```python
from build123d import *

# Parameters (mm, degrees)
F0_W     = 203.2
F0_H     = 76.2
F1_DEPTH = 76.708
F2_W     = 101.6
F2_H     = 38.1
F3_DEPTH = 116.332
F4_R     = 7.5946
F5_DEPTH = 234.95
F6_W     = 176.251258
F6_H     = 58.252844
F7_DEPTH = 93.472


with BuildPart() as f1:
    # F0 (on Front) → F1 (new body)
    with BuildSketch(Plane.XZ):
        with Locations((48.921661, 38.1)):
            Rectangle(F0_W, F0_H)
    extrude(amount=F1_DEPTH)

    # F2 (on Front) → F3 (cut)
    with BuildSketch(Plane.XZ):
        with Locations((49.131309, 57.448106)):
            Rectangle(F2_W, F2_H)
    extrude(amount=F3_DEPTH, mode=Mode.SUBTRACT)

    # F4 (on face) → F5 (cut, symmetric)
    with BuildSketch(Plane(origin=(-52.678339, 0, 0), x_dir=(0, -1, 0), z_dir=(-1, 0, 0))):
        with Locations((40.342383, 40.232584)):
            Circle(F4_R)
    extrude(amount=F5_DEPTH, both=True, mode=Mode.SUBTRACT)

    # F6 (on face) → F7 (cut)
    with BuildSketch(Plane(origin=(0, 0, 0), x_dir=(1, 0, 0), z_dir=(0, 0, -1))):
        with Locations((45.208322, 38.419208)):
            Rectangle(F6_W, F6_H)
    extrude(amount=-F7_DEPTH, mode=Mode.SUBTRACT)


solid = f1.part
```
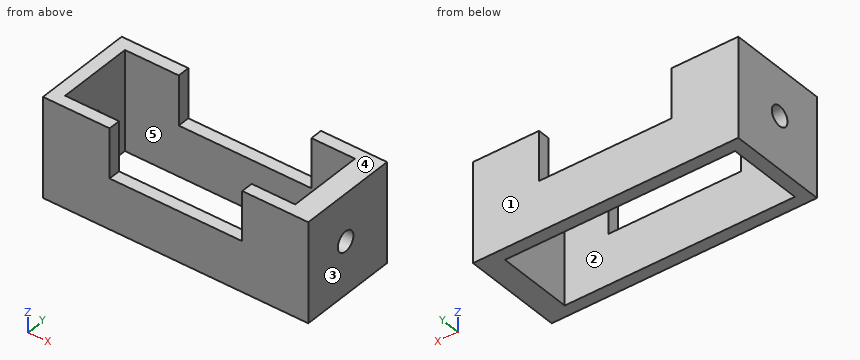
Can you work these out from the model? Positions are in its coordinate system, mm. Face numbers are marked on the shaded views. A direction names the side the tool comes from. Round coordinates to 2 decimals unless told otherwise and drop trailing zeros. Loops run counter-clockwise (first coordinate to the right, second up) from the corner with the lowest first, then second, coordinate; pieces in that order, holes last. Notation, with made-up numbers: M 36,5.25 L 88,5.25 A28 ccw 88,31.25 Z; hole C 69.5,-10 d9. An arc over 180 degrees is marked long. Answer as a JSON object with one key per item and string values. Group by question number.
Q1. Imagine slicing it at D-D, the plane y = -42. Please give me the cut outline in (x, z), then the cut area to 3 significant figures.
Q2. Will these pins go through, and if not, where does the flat tip stop? pin 1 (12 mm diameter, centred on y = -47, z = 39.5, fed in from -X); pin 2 (23 mm diameter, centred on x = 50.5, z = 50.5, fed in from +Y); pin 3 (10 mm diameter, centred on x = 32, y = -71, fed in from +Z).
Q3. Imagine slicing it at C-C, the plane y = -52.5. Please give me the cut outline in (x, z).
Q4. Please list where these lines run through material, in increasing order: L1, parallel to X at y = -61.5, z = 53.5; L2, parallel to Y at x = 31.5, z = 9.5; L3, parallel to X at y = -7, z = 58.
Q5. We'd pull the mould along X, two halves only. Please class the marked faces 3, 4 and 5: +X half, -X half, draft (parallel to the pull), parting line (faces both ways), or undercut.
Q6. Imagine slicing it at A-A, the plane z = 51.5. Please give me the cut outline in (x, y).
Q7. Imagine slicing it at B-B, the plane x = 78. Please give me the cut outline in (y, z), then the cut area to 3 significant figures.
Q8. On a 3-axis mill with a long thin cutter (end or side, diameter ignored), from which of +Z, -Z, +X, -X, +Y, -Y can I reach the whole of each face in a straight line? I mean the marked faces 1 and 2. Say none if no direction works.
Findings:
{
 "1": {"outline": "M -52.68,0 L -42.92,0 L -42.92,32.82 L -52.68,32.82 Z; M -52.68,47.64 L -42.92,47.64 L -42.92,76.2 L -52.68,76.2 Z; M 133.33,0 L 150.52,0 L 150.52,32.82 L 133.33,32.82 Z; M 133.33,47.64 L 150.52,47.64 L 150.52,76.2 L 133.33,76.2 Z", "area": "1,650 mm2"},
 "2": {"pin 1": "stops at x = -52.68", "pin 2": "passes through", "pin 3": "stops at z = 38.4"},
 "3": {"outline": "M -52.68,0 L -42.92,0 L -42.92,76.2 L -52.68,76.2 Z; M 133.33,0 L 150.52,0 L 150.52,76.2 L 133.33,76.2 Z"},
 "4": {"L1": "x = -52.68 to -42.92, 133.33 to 150.52", "L2": "y = -76.71 to -67.55, -9.29 to 0", "L3": "x = -52.68 to -1.67, 99.93 to 150.52"},
 "5": {"face 3": "+X half", "face 4": "draft", "face 5": "undercut"},
 "6": {"outline": "M -52.68,-76.71 L -1.67,-76.71 L -1.67,-67.55 L -42.92,-67.55 L -42.92,-9.29 L -1.67,-9.29 L -1.67,0 L -52.68,0 Z; M 99.93,-76.71 L 150.52,-76.71 L 150.52,0 L 99.93,0 L 99.93,-9.29 L 133.33,-9.29 L 133.33,-67.55 L 99.93,-67.55 Z"},
 "7": {"outline": "M -76.71,0 L -67.55,0 L -67.55,38.4 L -76.71,38.4 Z; M -9.29,0 L 0,0 L 0,38.4 L -9.29,38.4 Z", "area": "709 mm2"},
 "8": {"face 1": "+Z, -Z, +X, -X, +Y", "face 2": "+Z, -Z"}
}
